Part model, mm, in its own coordinate system. Face numbers are marked on the shaded views. A direction names the side the tool comes from. Coordinates: 2 decimals unless noted, no trailing zeros. Write each loop counter-clockwise with the first axis right and the second up, starting at its lowest first coordinate (ties: lowest second). Pieces come first, ordered by that corner, then holes. Notation, with made-up numbers: (28.5, 39) -> (53.5, 39) arc R15 cw to (53.5, 51) -> close; hole circle Ø2 at (12.5, -38.75). An arc over 180 degrees is marked (long way). Write item = value, one per line.
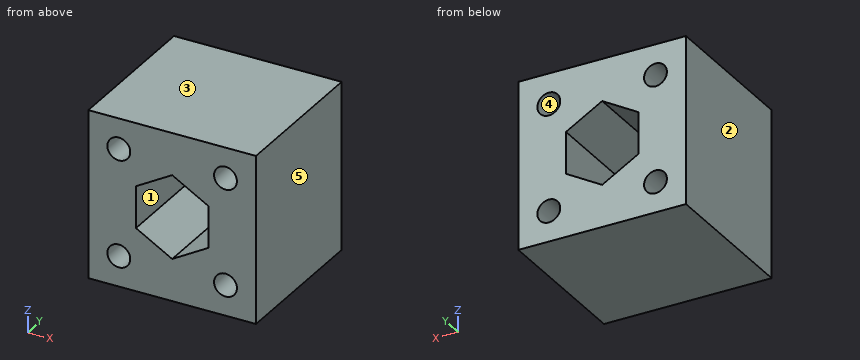
from build123d import *

# Parameters (mm, degrees)
F0_W     = 44
F0_H     = 44
F0_R     = 3
F1_DEPTH = 20


with BuildPart() as f1:
    # F0 (on Front) → F1 (new body, symmetric)
    with BuildSketch(Plane.XZ):
        Rectangle(F0_W, F0_H)
        with Locations((-14, -14)):
            Circle(F0_R, mode=Mode.SUBTRACT)
        with Locations((14, -14)):
            Circle(F0_R, mode=Mode.SUBTRACT)
        with Locations((-14, 14)):
            Circle(F0_R, mode=Mode.SUBTRACT)
        Polygon((0, 10.9696551146), (9.5, 5.4848275573), (9.5, -5.4848275573), (0, -10.9696551146), (-9.5, -5.4848275573), (-9.5, 5.4848275573), align=None, mode=Mode.SUBTRACT)
        with Locations((14, 14)):
            Circle(F0_R, mode=Mode.SUBTRACT)
    extrude(amount=F1_DEPTH, both=True)


solid = f1.part
Q1. Saw through at D-D on z = 3. Give the cut face in (x, y).
Model answer:
outline = (-22, -20) -> (-9.5, -20) -> (-9.5, 20) -> (-22, 20) -> close; (9.5, -20) -> (22, -20) -> (22, 20) -> (9.5, 20) -> close
Q2. Pin check, flat tips, straight feed: pin 1 (5 mm diameter, centred on x = -14, z = -14, fed in from -Y); pin 2 (8 mm diameter, centred on x = 14, z = -14, fed in from +Y). Stop position of each tip, or through.
Model answer:
pin_1 = through
pin_2 = 20
Q3. Saw through at C-C on y = 6. Give the cut face in (x, z).
Model answer:
outline = (-22, -22) -> (22, -22) -> (22, 22) -> (-22, 22) -> close; hole circle Ø6 at (-14, -14); hole circle Ø6 at (-14, 14); hole (-9.5, -5.48) -> (0, -10.97) -> (9.5, -5.48) -> (9.5, 5.48) -> (0, 10.97) -> (-9.5, 5.48) -> close; hole circle Ø6 at (14, -14); hole circle Ø6 at (14, 14)
Q4. Mould opens along X. For the marked faces 3, 4 and 5 say: released by +X, released by -X, zero draft, split by the parting line, or undercut.
Model answer:
face_3 = zero draft
face_4 = undercut
face_5 = released by +X
Q5. Saw through at B-B on z = 14. Give the cut face in (x, y), and give its area (3 significant figures).
Model answer:
outline = (-22, -20) -> (-17, -20) -> (-17, 20) -> (-22, 20) -> close; (-11, -20) -> (11, -20) -> (11, 20) -> (-11, 20) -> close; (17, -20) -> (22, -20) -> (22, 20) -> (17, 20) -> close
area = 1,280 mm²
Q6. Which spindle directions (+Z, -Z, +X, -X, +Y, -Y) get a long thin tool onto all of the face, cutting with end or side? Do the marked faces 1 and 2. Say none if no direction does.
Model answer:
face_1 = +Y, -Y
face_2 = +Z, -Z, -X, +Y, -Y
Q7. Probe line 1 (Z direction, x = -14, y = -7); line 2 (X direction, y = 7, z = -3); line 3 (X direction, y = -13, z = -13). List the from-to ranges inside material, lowest first. Write a range as from..to.
Model answer:
line_1 = -22..-17, -11..11, 17..22
line_2 = -22..-9.5, 9.5..22
line_3 = -22..-16.83, -11.17..11.17, 16.83..22
Q8. Saw through at A-A on x = -14. Give the cut face in (y, z).
Model answer:
outline = (-20, -22) -> (20, -22) -> (20, -17) -> (-20, -17) -> close; (-20, -11) -> (20, -11) -> (20, 11) -> (-20, 11) -> close; (-20, 17) -> (20, 17) -> (20, 22) -> (-20, 22) -> close
